Geometry check sheet. Reference: drawing and pictorial views, mm from the part's lowest x, y, z. A direction names the side the tool comes from. Give positions to 0.01 mm unless a question says otherwise; leave off trailing zeros. Write each loop counter-clockwise with the first axis right and the second up, starting at its lowest first coordinate (ties: lowest second). Pieces come first, ordered by that corner, then holes. Notation, with made-up numbers: (-33.75, 20.25) -> (21.25, 20.25) arc R24 cw to (21.25, 57.25) -> close; hole circle Ø2 at (38.5, 13). An arc over 180 degrees is marked (long way). Use a Markdown table: item, result. Add a question column.
1. Cross-section at A-A (z = 2). Enter the section's corners in (x, y).
2. Cross-section at C-C (x = 15.75). Enter the section's corners in (y, z), then the cut area to 3 significant figures.
3. Scan lines: probe 1 along X at (y, z) = (36, 5.75); probe 2 along Z at (x, y) = (22, 31); probe 3 along Z at (x, y) = (28, 34). Record each from-to range of solid material in increasing order. Write a range as [from, to].
4. Set-up check for the marked faces 5, 6 and 7: record each of +Z, -Z, +X, -X, +Y, -Y from which the full face is reachable in a straight line by a thin tool's end or side.
5. Gauge pin test, flat ends, axial feed: P1, Ø4, axis at y = 38, z = 4, coming from the -X side; P2, Ø8, axis at x = 9.5, y = 28.5, coming from the +Z side; P3, Ø1.5, axis at x = 8, y = 15.5, coming from the -Z side. Record the tip position at first contact, or that the pin passes through.
6. Release check for a two-part mould opening along X. For the marked faces 1, 2, 3 and 4 record: released by +X, released by -X, zero draft, split by the parting line, or undercut.
7. Cross-section at D-D (y = 14). Enter the section's corners in (x, z).
8. Cross-section at B-B (y = 28). Enter the section's corners in (x, z).
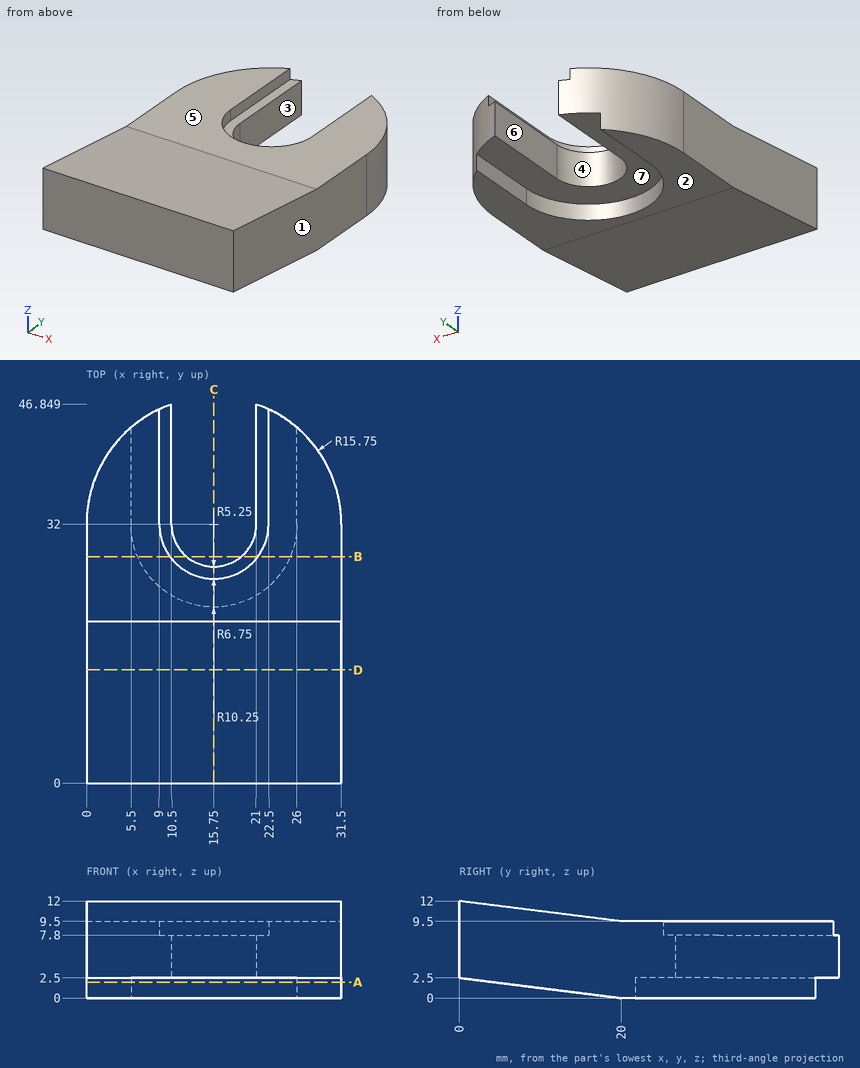
Worked answers:
| question | item | result |
|---|---|---|
| 1 | outline | (0, 4) -> (31.5, 4) -> (31.5, 32) arc R15.75 ccw to (26, 43.96) -> (26, 32) arc R10.25 cw to (5.5, 32) -> (5.5, 43.96) arc R15.75 ccw to (0, 32) -> close |
| 2 | outline | (0, 2.5) -> (20, 0) -> (21.75, 0) -> (21.75, 2.5) -> (26.75, 2.5) -> (26.75, 7.8) -> (25.25, 7.8) -> (25.25, 9.5) -> (20, 9.5) -> (0, 12) -> close |
| 2 | area | 239 mm² |
| 3 | probe 1 | x = [0.52, 10.5], [21, 30.98] |
| 3 | probe 2 | z = [2.5, 7.8] |
| 3 | probe 3 | z = [0, 9.5] |
| 4 | face 5 | +Z, +X, -X, +Y |
| 4 | face 6 | +Z, -Z, +Y |
| 4 | face 7 | -Z, +Y |
| 5 | P1 | stops at x = 0.52 |
| 5 | P2 | stops at z = 9.5 |
| 5 | P3 | stops at z = 0.47 |
| 6 | face 1 | released by +X |
| 6 | face 2 | zero draft |
| 6 | face 3 | undercut |
| 6 | face 4 | undercut |
| 7 | outline | (0, 0.75) -> (31.5, 0.75) -> (31.5, 10.25) -> (0, 10.25) -> close |
| 8 | outline | (0, 0) -> (6.31, 0) -> (6.31, 2.5) -> (12.35, 2.5) -> (12.35, 7.8) -> (10.31, 7.8) -> (10.31, 9.5) -> (0, 9.5) -> close; (19.15, 2.5) -> (25.19, 2.5) -> (25.19, 0) -> (31.5, 0) -> (31.5, 9.5) -> (21.19, 9.5) -> (21.19, 7.8) -> (19.15, 7.8) -> close |
